Geometry: final body of the model. Coordinates: model frame, mm. Give positions to 0.01 mm unless a question says otherwise; leave off trailing zeros. Loops run counter-clockwise (first coordinate to the right, second up) from the corner with the lowest first, then second, coordinate; pieces in that order, holes last. Notation, with made-up numbers: (14.5, -16.5) -> (24.5, -16.5) arc R22 ccw to (24.5, 10.5) -> close; hole circle Ø1 at (44, 67.25). An arc over 180 degrees is marked (long way). Answer in a Markdown table with one row per item. Add a question column.
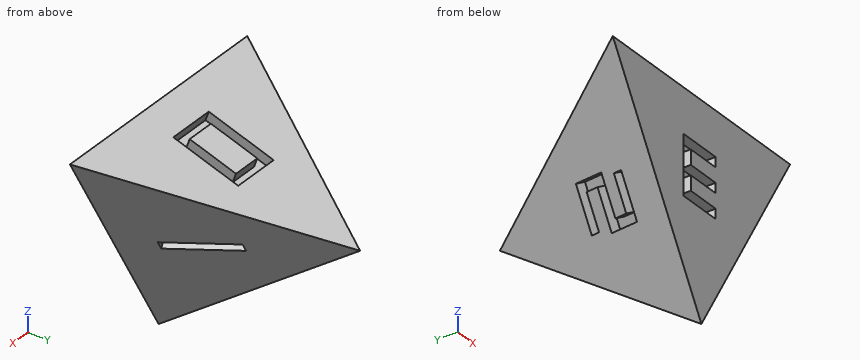
from build123d import *

# Parameters (mm, degrees)
SKETCH4_W               = 0.254
SKETCH4_H               = 0.254
CUT_EXTRUDE1_DEPTH      = 0.508
CUT_EXTRUDE2_DEPTH      = 0.508
CUT_EXTRUDE3_DEPTH      = 0.508
CUT_EXTRUDE4_DEPTH      = 1.0000001
CUT_EXTRUDE4_DEPTH_BACK = 0.508


with BuildPart() as part:
    # Sketch1 → Loft1 section 0
    with BuildSketch(Plane(origin=(0, 0, 0), x_dir=(1, 0, 0), z_dir=(0, 1, 0)), mode=Mode.PRIVATE) as loft1_s0:
        Polygon((0, 7.332348419), (-6.35, -3.666174209), (6.35, -3.666174209), align=None)
    loft([Vertex(0, 10.414, 0), loft1_s0.sketch])

    # Sketch4 → Cut-Extrude1 (cut)
    with BuildSketch(Plane(origin=(0, 1.148332745, 3.26191188), x_dir=(1, 0, 0), z_dir=(0, 0.332066518, 0.943255972))):
        Polygon((-1.27, 0.560586297), (1.27, 0.560586297), (1.27, 2.338586297), (1.27, 4.116586297), (-1.27, 4.116586297), (-1.27, 2.338586297), align=None)
        Polygon((1.016, 0.814586297), (1.016, 2.338586297), (1.016, 3.862586297), (-1.016, 3.862586297), (-1.016, 2.338586297), (-1.016, 0.814586297), align=None, mode=Mode.SUBTRACT)
        Polygon((-1.016, 3.862586297), (-1.016, 2.592586297), (-0.762, 2.592586297), (-0.762, 3.608586297), (0.762, 3.608586297), (0.762, 2.592586297), (1.016, 2.592586297), (1.016, 3.862586297), align=None)
        with Locations((-0.889, 2.465586297)):
            Rectangle(SKETCH4_W, SKETCH4_H)
        with Locations((-0.889, 2.211586297)):
            Rectangle(SKETCH4_W, SKETCH4_H)
        Polygon((-0.762, 2.084586297), (-1.016, 2.084586297), (-1.016, 0.814586297), (1.016, 0.814586297), (1.016, 2.084586297), (0.762, 2.084586297), (0.762, 1.068586297), (-0.762, 1.068586297), align=None)
        with Locations((0.889, 2.465586297)):
            Rectangle(SKETCH4_W, SKETCH4_H)
        with Locations((0.889, 2.211586297)):
            Rectangle(SKETCH4_W, SKETCH4_H)
    extrude(amount=-CUT_EXTRUDE1_DEPTH, mode=Mode.SUBTRACT)

    # Sketch6 → Cut-Extrude2 (cut)
    with BuildSketch(Plane(origin=(2.824898553, 1.148332745, -1.63095594), x_dir=(-0.436908848, -0.177605223, -0.88179762), z_dir=(0.816883634, 0.332066518, -0.471627986))):
        Polygon((-1.120218022, 4.494043391), (-0.402834916, 0.752190711), (0.096078775, 0.847841792), (-0.621304332, 4.589694472), align=None)
    extrude(amount=-CUT_EXTRUDE2_DEPTH, mode=Mode.SUBTRACT)

    # Sketch7 → Cut-Extrude3 (cut)
    with BuildSketch(Plane(origin=(-2.824898553, 1.148332745, -1.63095594), x_dir=(-0.436908848, 0.177605223, 0.88179762), z_dir=(-0.816883634, 0.332066518, -0.471627986))):
        Polygon((1.246856533, 1.10762778), (1.151205452, 0.60871409), (-1.093906156, 1.039143954), (-0.759127373, 2.785341871), (1.23652739, 2.402737547), (1.380004011, 3.151108083), (-0.366193906, 3.485886867), (-0.270542826, 3.984800557), (1.974568782, 3.554370693), (1.639789999, 1.808172776), (-0.355864763, 2.190777099), (-0.499341385, 1.442406563), align=None)
    extrude(amount=-CUT_EXTRUDE3_DEPTH, mode=Mode.SUBTRACT)

    # Sketch8 → Cut-Extrude4 (cut, two sides)
    with BuildSketch(Plane.XZ) as cut_extrude4_sk:
        Polygon((-0.762, 0.872174209), (1.016, 0.872174209), (1.016, 1.380174209), (-1.27, 1.380174209), (-1.27, -1.667825791), (1.016, -1.667825791), (1.016, -1.159825791), (-0.762, -1.159825791), (-0.762, -0.397825791), (1.016, -0.397825791), (1.016, 0.110174209), (-0.762, 0.110174209), align=None)
    extrude(amount=CUT_EXTRUDE4_DEPTH, mode=Mode.SUBTRACT)
    extrude(cut_extrude4_sk.sketch, amount=-CUT_EXTRUDE4_DEPTH_BACK, mode=Mode.SUBTRACT)


solid = part.part
(1) Pin query (flat end, axial travel): pin 1 Ø1.1 at (y, z) = (3, 2) entering from +X; pin 2 Ø1.3 at (y, z) = (3, 2) entering from -X; pin 3 Ø0.6 at (y, z) = (0, 1) entering from -X; pin 4 Ø1.5 at (x, z) = (3.5, -5.5) entering from +Y. Return the tip coordinate at first contact, or that it passes through.
(2) Cut plane A-A on y = 2.75. Return the cut outline in (x, z), then the cut area to 3 significant figures.
(3) Material intervals for line 1 along Y through (x, z) = (-2, 0); line 2 along X through (y, z) = (2, -1.5); line 3 along Y through (x, z) = (1.75, 0.5), sorted ascending. Write a range as from..to.
(4) Cut plane C-C on x = -4.25. Return the cut outline in (y, z).
(5) Cut plane B-B on z = -3.5. Return the cut outline in (x, y), then the cut area to 3 significant figures.
Answer list:
| question | item | result |
|---|---|---|
| 1 | pin 1 | stops at x = 4.56 |
| 1 | pin 2 | stops at x = -4.63 |
| 1 | pin 3 | stops at x = -4.98 |
| 1 | pin 4 | passes through |
| 2 | outline | (-4.67, 2.7) -> (-1.96, -2.01) -> (-1.49, -1.74) -> (-1.24, -2.18) -> (-1.7, -2.45) -> (0, -5.4) -> (2.21, -1.57) -> (1.74, -1.3) -> (2, -0.86) -> (2.46, -1.13) -> (4.67, 2.7) -> (1.27, 2.7) -> (1.27, 2.16) -> (0.76, 2.16) -> (0.76, 2.7) -> (-0.76, 2.7) -> (-0.76, 2.16) -> (-1.27, 2.16) -> (-1.27, 2.7) -> close |
| 2 | area | 36.7 mm² |
| 3 | line 1 | y = 0..3.96, 4.7..5.49 |
| 3 | line 2 | x = -1.93..2.09 |
| 3 | line 3 | y = 0..6.82 |
| 4 | outline | (0, 0.03) -> (3.44, 2.45) -> (0, 3.67) -> close |
| 5 | outline | (-2.21, 0) -> (2.21, 0) -> (0, 5.44) -> close |
| 5 | area | 12.0 mm² |
